Print and shaded views of the part. All mm, measured from the part's lowest x, y and z. A direction names the side the tool comes from. Coordinates: 2 decimals unless noted, no trailing zeros. Write each loop counter-clockwise with the first axis right and the second up, starting at its lowest first coordinate (ties: lowest second). Pieces come first, ordered by that corner, then holes. Notation, with made-up numbers: (19, 2.25) -> (52, 2.25) arc R21 cw to (52, 9.25) -> close; hole circle Ø11 at (26.5, -6.75). An arc over 180 degrees is marked (long way). Write item = value, one per line.
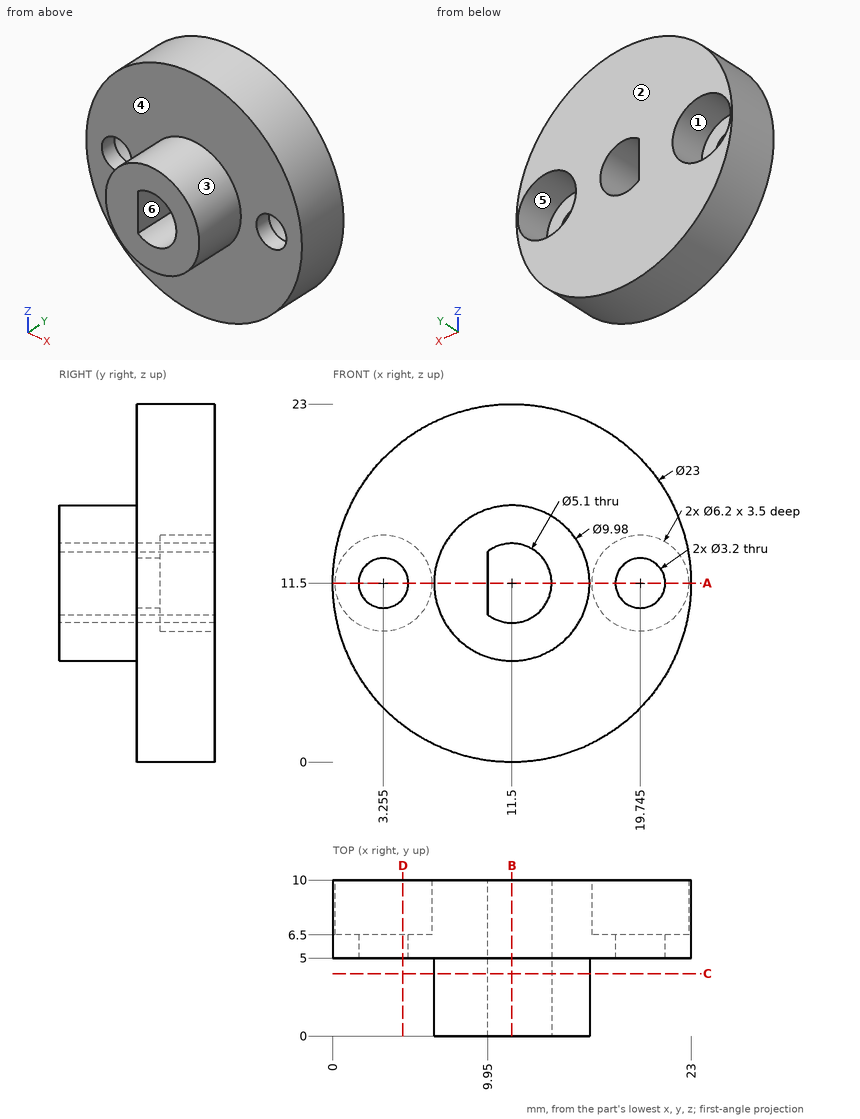
Q1. Saw through at C-C on y = 4. Give the cut face in (x, z), and give its area (3 significant figures).
Model answer:
outline = circle Ø9.98 at (11.5, 11.5); hole (9.95, 9.48) arc R2.55 ccw (long way) to (9.95, 13.52) -> close
area = 60.6 mm²
Q2. Mould opens along X. For the marked faces 3, 4, 5 and 6 say: released by +X, released by -X, zero draft, split by the parting line, or undercut.
Model answer:
face_3 = split by the parting line
face_4 = zero draft
face_5 = undercut
face_6 = undercut
Q3. Saw through at B-B on x = 11.5. Give the cut face in (y, z).
Model answer:
outline = (0, 6.51) -> (5, 6.51) -> (5, 0) -> (10, 0) -> (10, 8.95) -> (0, 8.95) -> close; (0, 14.05) -> (10, 14.05) -> (10, 23) -> (5, 23) -> (5, 16.49) -> (0, 16.49) -> close
Q4. Pin check, flat tips, straight feed: pin 1 (1.9 mm diameter, centred on x = 2.5, z = 12.5, fed in from +Y); pin 2 (4 mm diameter, centred on y = 6, z = 20.5, fed in from +X); pin 3 (6 mm diameter, centred on x = 8.5, y = 3.5, fed in from -Z). Stop position of each tip, or through.
Model answer:
pin_1 = 6.5
pin_2 = 20.62
pin_3 = 0.01
Q5. Saw through at A-A on z = 11.5. Give the cut face in (x, y) (3 decimals).
Model answer:
outline = (0, 5) -> (1.655, 5) -> (1.655, 6.5) -> (0.155, 6.5) -> (0.155, 10) -> (0, 10) -> close; (4.855, 5) -> (6.51, 5) -> (6.51, 0) -> (9.95, 0) -> (9.95, 10) -> (6.355, 10) -> (6.355, 6.5) -> (4.855, 6.5) -> close; (14.05, 0) -> (16.49, 0) -> (16.49, 5) -> (18.145, 5) -> (18.145, 6.5) -> (16.645, 6.5) -> (16.645, 10) -> (14.05, 10) -> close; (21.345, 5) -> (23, 5) -> (23, 10) -> (22.845, 10) -> (22.845, 6.5) -> (21.345, 6.5) -> close
Q6. Which spindle directions (+Z, -Z, +X, -X, +Y, -Y) get a long thin tool onto all of the face, cutting with end or side? Do the marked faces 1 and 2. Say none if no direction does.
Model answer:
face_1 = +Y
face_2 = +Z, -Z, +X, -X, +Y
Q7. Probe line 1 (X direction, y = 7.85, z = 11.5) (3 decimals); line 2 (X direction, y = 8.25, z = 10.5); line 3 (Z direction, x = 11.5, y = 2.75). List the from-to ranges inside material, lowest first. Write a range as from..to.
Model answer:
line_1 = 0..0.155, 6.355..9.95, 14.05..16.645, 22.845..23
line_2 = 0.04..0.32, 6.19..9.95, 13.85..16.81, 22.68..22.96
line_3 = 6.51..8.95, 14.05..16.49
Q8. Saw through at D-D on x = 4.5. Give the cut face in (y, z), and give its area (3 significant figures).
Model answer:
outline = (5, 2.38) -> (10, 2.38) -> (10, 8.66) -> (6.5, 8.66) -> (6.5, 10.5) -> (5, 10.5) -> close; (5, 12.5) -> (6.5, 12.5) -> (6.5, 14.34) -> (10, 14.34) -> (10, 20.62) -> (5, 20.62) -> close
area = 68.4 mm²
